Design review of the part built by this model. Coordinates are the model's own, in mm. Face numbers are marked on the shaded views. A direction names the side the tool comes from. Round coordinates to 2 decimals unless told otherwise and drop trailing zeros. Order: outer loops, then holes, each group sorted by start corner. A loop starts at its lowest first (then second) coordinate and runs counter-clockwise, first axis right, second up. Notation, with made-up numbers: (31.25, -17.75) - (39.25, -17.75) arc R29 ccw to (39.25, 11.25) - close; hole circle Ø3 at (-3, -37.75). An arc over 180 degrees is marked (long way). Write item = value, one per line.
from build123d import *

# Parameters (mm, degrees)
F1_DEPTH = 63.5
F0_W     = 25.4
F0_H     = 19.05
F2_DEPTH = 25.4
F3_DEPTH = 8.255


with BuildPart() as f1:
    # F0 (on Front) → F1 (new body, symmetric)
    with BuildSketch(Plane.XZ):
        Polygon((-41.275, 9.525), (-41.275, -9.525), (41.275, -9.525), (41.275, 9.525), (22.225, 9.525), align=None)
    extrude(amount=F1_DEPTH, both=True)

    # F0 (on Front) → F2 (join, symmetric)
    with BuildSketch(Plane.XZ):
        with BuildLine():
            Line((22.225, 9.525), (41.275, 9.525))
            Line((41.275, 9.525), (41.275, 27.0002))
            ThreePointArc((41.275, 27.0002), (45.9246798487, 38.2255201513), (57.15, 42.8752))
            Line((57.15, 42.8752), (60.325, 42.8752))
            Line((60.325, 42.8752), (60.325, 61.9252))
            Line((60.325, 61.9252), (57.15, 61.9252))
            ThreePointArc((57.15, 61.9252), (32.4542956671, 51.6959043329), (22.225, 27.0002))
            Line((22.225, 27.0002), (22.225, 9.525))
        make_face()
        with Locations((73.025, 52.4002)):
            Rectangle(F0_W, F0_H)
    extrude(amount=F2_DEPTH, both=True)

    # F0 (on Front) → F3 (join, symmetric)
    with BuildSketch(Plane.XZ):
        with BuildLine():
            add(Edge.make_bspline(
                [(-41.275, 9.525), (-50.8186854422, 45.0256727636), (2.9303120675, 71.7999846045), (57.15, 61.9252)],
                knots=[0, 0, 0, 0, 111.5045361635, 111.5045361635, 111.5045361635, 111.5045361635], degree=3))
            Line((-41.275, 9.525), (22.225, 9.525))
            Line((22.225, 9.525), (22.225, 27.0002))
            ThreePointArc((22.225, 27.0002), (32.4542956671, 51.6959043329), (57.15, 61.9252))
        make_face()
    extrude(amount=F3_DEPTH, both=True)

    # F0 (on Front) → F4 (revolve)
    with BuildSketch(Plane.XZ):
        Polygon((85.725, 66.675), (85.725, 61.9252), (85.725, 42.8752), (85.725, 38.1), (111.125, 38.1), (111.125, 66.675), align=None)
    revolve(axis=Axis((85.725, 0, 52.3875), (0, 0, -1)))


solid = f1.part
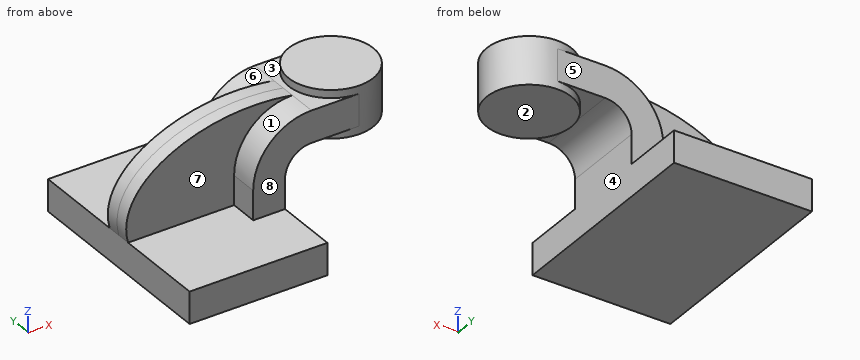
1) We need section C-C on x = 95.5. Write out the cut boundary in (y, z) (3 decimals), and give its area (3 significant figures).
Findings:
outline = (-23.444, 38.1) - (23.444, 38.1) - (23.444, 66.675) - (-23.444, 66.675) - close
area = 1,340 mm^2
2) The part is to be moulded in two halves that separate along X. For the marked faces 1, 2, 3 and 4, say which applies: released by +X, released by -X, zero draft, split by the parting line, or undercut.
Findings:
face_1 = released by -X
face_2 = zero draft
face_3 = undercut
face_4 = released by +X
3) We need section B-B on z = 5. Write out the cut boundary in (x, y) (3 decimals), and give its area (3 significant figures).
Findings:
outline = (-41.275, -63.5) - (41.275, -63.5) - (41.275, 63.5) - (-41.275, 63.5) - close
area = 10,500 mm^2
4) We need section A-A on y = 19.5. Write out the cut boundary in (x, z) (3 decimals), and give its area (3 significant figures).
Findings:
outline = (-41.275, -9.525) - (41.275, -9.525) - (41.275, 27) arc R15.875 cw to (57.15, 42.875) - (69.449, 42.875) - (69.449, 38.1) - (102.001, 38.1) - (102.001, 66.675) - (69.449, 66.675) - (69.449, 61.925) - (57.15, 61.925) arc R34.925 ccw to (22.225, 27) - (22.225, 9.525) - (-41.275, 9.525) - close
area = 3,830 mm^2
5) Clearance check with flat-ended pins moving along their axes: pin 1 Ø12 at (x, y) = (81, 4) entering from -Z; pin 2 Ø8.5 at (y, z) = (-16.5, 16) entering from -X (3 decimals); pin 3 Ø1 at (x, z) = (83, 36) entering from -Y; pin 4 Ø6 at (x, z) = (54, 59) entering from +Y. State where each tip first meets the part, or that it passes through.
Findings:
pin_1 = 38.1
pin_2 = 22.225
pin_3 = through
pin_4 = 25.4
6) For the marked faces 5, 6, 7 and 8, list the 3-axis set-ups (+Z, -Z, +X, -X, +Y, -Y) from which the entire face can be reached by the end or side of a thin tool; tool diameter is ignored.
Findings:
face_5 = +Z, +X, -X, +Y
face_6 = +Z, -X, +Y
face_7 = +Z, -X, -Y
face_8 = +Z, +X, -X, -Y
7) To check wall thickness, follow L1, parallel to Y at x = -27, z = 20.5 (3 decimals); L2, parallel to X at y = 45, z = 0 (3 decimals); L3, parallel to Y at x = 25, z = 24. State the ranges of each line that lie inside material, in increasing order. Write a range as from..to.
Findings:
L1 = -8.255..8.255
L2 = -41.275..41.275
L3 = -25.4..25.4
